Model file for the job. Use its own axes, mm. Face numbers are marked on the shaded views. A direction names the side the tool comes from. Coordinates: 2 decimals unless noted, no trailing zeros. Write each loop counter-clockwise with the first axis right and the second up, starting at its lowest first coordinate (ties: lowest second). Pieces come first, ordered by that corner, then holes. Notation, with made-up numbers: M 75,58.5 L 79,58.5 A29 ccw 79,97.5 Z; hole C 12,-1 d7. An arc over 180 degrees is marked long. Answer in a Markdown table with one row per item. Add a question column.
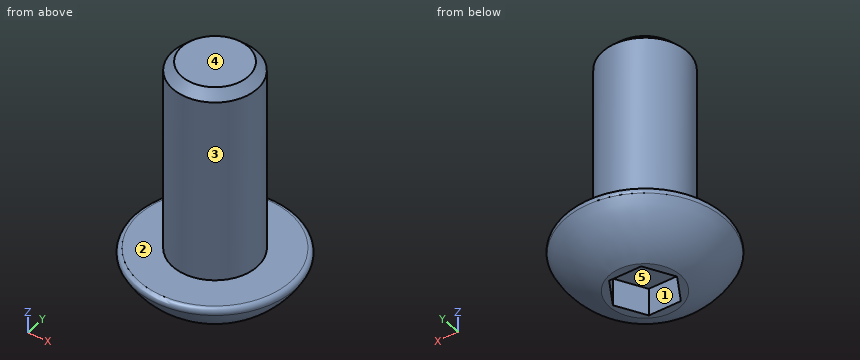
Autodesk Inventor part; units mm, degrees
ref_plane "YZ Plane" through (0, 0, 0) normal (1, 0, 0) x (0, 1, 0)
ref_plane "XZ Plane" through (0, 0, 0) normal (0, 1, 0) x (-1, 0, 0)
ref_plane "XY Plane" through (0, 0, 0) normal (0, 0, 1) x (1, 0, 0)
sketch "Sketch1" plane through (0, 0, 0) normal (0, 0, 1) x (1, 0, 0)
  circle A0 centre (0, 0) radius 2.413
  dimension "d0" = 4.826
extrude "Extrusion1" add sketch "Sketch1" along normal blind 11.1125
sketch "Sketch2" plane through (0, 0, 0) normal (0, 1, 0) x (-1, 0, 0)
  line L0 (0, 0) -> (0, -2.5654)
  line L1 (0, 0) -> (4.3239, 0)
  line L2 (0, -2.5654) -> (2.032, -2.5654)
  line L3 (4.3239, 0) -> (4.3239, 3.8864) construction
  arc A0 (4.5568, -0.3781) -> (4.3239, 0) centre (4.3239, -0.2608) ccw
  arc A1 (2.032, -2.5654) -> (4.5568, -0.3781) centre (0.6382, 1.5944) ccw
  line L4 (4.5847, 0.6553) -> (4.5847, -0.2608) construction
  dimension "d3" = 2.5654
  dimension "d6" = 2.032
  dimension "d12" = 4.5847
revolve "Revolution1" add sketch "Sketch2" angle 360 about axis through (0, 0, 0) along (0, 0, -1)
sketch "Sketch3" plane through (0, 0, -2.5654) normal (0, 0, -1) x (-1, 0, 0)
  circle A0 centre (0, 0) radius 2.032
  line L0 (-0.9165, 1.5875) -> (0.9165, 1.5875)
  line L1 (0.9165, 1.5875) -> (1.8331, 0)
  line L2 (1.8331, 0) -> (0.9165, -1.5875)
  line L3 (0.9165, -1.5875) -> (-0.9165, -1.5875)
  line L4 (-0.9165, -1.5875) -> (-1.8331, 0)
  line L5 (-1.8331, 0) -> (-0.9165, 1.5875)
  dimension "d8" = 3.175
extrude "Extrusion2" cut sketch "Sketch3" against normal blind 1.5875 contours L0 L1 L2 L3 L4 L5
chamfer "Chamfer1" distance 0.508 angle 45 1 edges at (-2.413, 0, 11.1125)
thread "Thread1"
properties part number "10-32 x438 button head" material "Steel"
1) Two-plate mould, pull along Y, no slides. Class the marked faces 1, 2 and 3: released by +Y, released by -Y, zero draft, split by the parting line, or undercut.
2) Flat gauge pins, fed straight in: pin 1 Ø1.3 at (x, z) = (0, -1.5) entering from +Y; pin 2 Ø0.8 at (x, z) = (0, -2) entering from -Y; pin 3 Ø1 at (x, z) = (0.5, 2) entering from -Y. Where does each tip first touch, or does it go through?
3) Drill centre lines: probe 1 along Y at (x, z) = (0, 1.5); probe 2 along Y at (x, z) = (2, 2.75); probe 3 along Z at (x, y) = (-0.75, 0). Where is each one in solid material? Low to high.
4) Which spindle directions (+Z, -Z, +X, -X, +Y, -Y) get a long thin tool onto all of the face, cutting with end or side? Do the marked faces 4 and 5. Say none if no direction does.
5) Slice it at A-A (z = 9.5). Give the cut face in (x, y).
Ans:
| question | item | result |
|---|---|---|
| 1 | face 1 | undercut |
| 1 | face 2 | zero draft |
| 1 | face 3 | split by the parting line |
| 2 | pin 1 | stops at y = 4.28 |
| 2 | pin 2 | stops at y = -3.65 |
| 2 | pin 3 | stops at y = -2.41 |
| 3 | probe 1 | y = -2.41 to 2.41 |
| 3 | probe 2 | y = -1.35 to 1.35 |
| 3 | probe 3 | z = -0.98 to 11.11 |
| 4 | face 4 | +Z, +X, -X, +Y, -Y |
| 4 | face 5 | -Z |
| 5 | outline | C 0,0 d4.83 |
